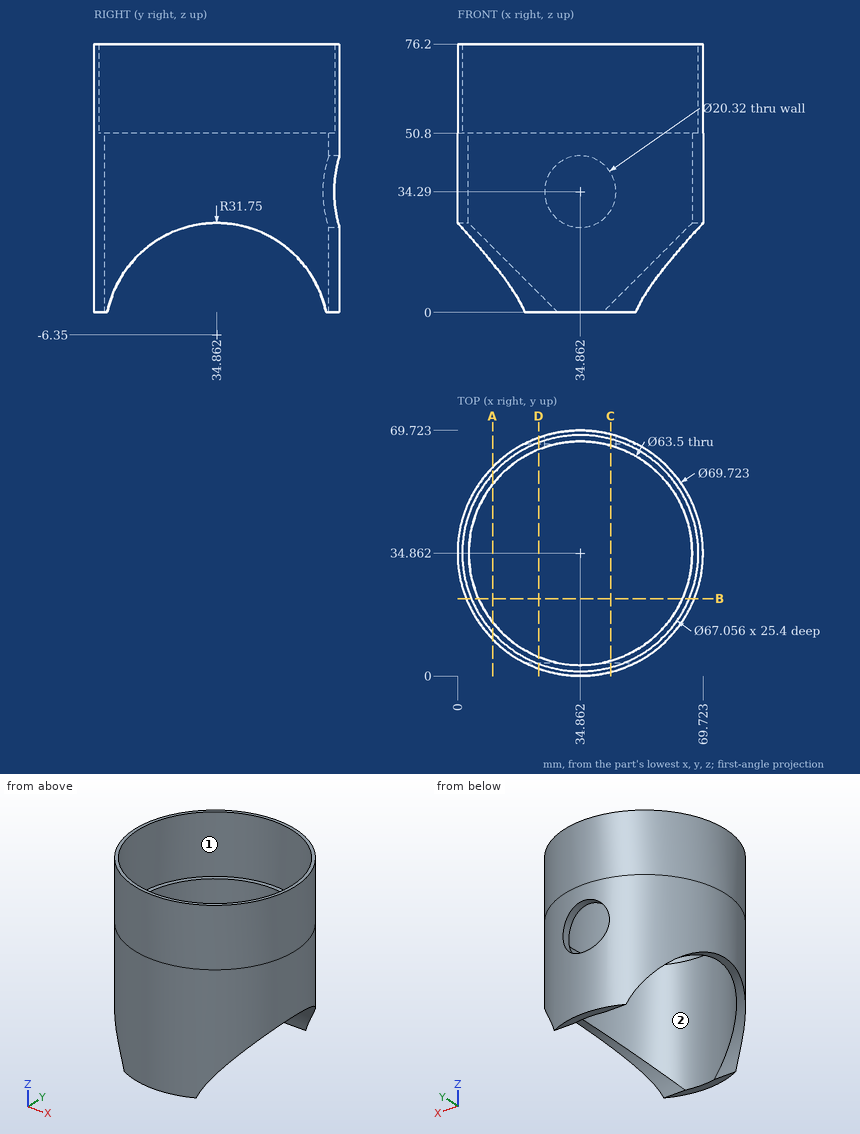
Source: three-view drawing plus pictorial views. Frame: mm from the lowest corner of the part. A direction names the side the tool comes from. Give positions to 0.01 mm unless a question says otherwise; leave off trailing zeros. Order: outer loops, then holes, each group sorted by start corner. A loop starts at its lowest first (then second) coordinate and runs counter-clockwise, first axis right, second up. Notation, with made-up numbers: (39, -37.5) - (88, -37.5) arc R29 ccw to (88, -14.5) - close; hole circle Ø5 at (23, 33). An arc over 180 degrees is marked (long way). Answer as a JSON object with one key per item and string values. Group by question number.
Q1. Set-up query: the marked faces 1 and 2. Return all of +Z, -Z, +X, -X, +Y, -Y with unobstructed straight access to the full face (end or side cutting, diameter ignored); none if empty.
Q2. Cut plane A-A, the plane x = 10. Output: boundary loops of the cut face in (y, z).
Q3. First-contact query: pin 1 Ø10 at (x, z) = (17, 18) entering from -Y; pin 2 Ø5 at (y, z) = (48.5, 42) entering from -X; pin 3 Ø12 at (x, z) = (34.86, 34.29) entering from -Y. Flat tips, straight axial feed; report the tip coordinate or a pass-through.
Q4. Cut plane D-D, the plane x = 23. Output: boundary loops of the cut face in (y, z).
Q5. Cut plane C-C, the plane x = 43.5. Count the separate pieces of the cut face and the enclosed holes in it.
Q6. Line query: probe 1 along X at (y, z) = (53.5, 63.5); probe 2 along Y at (x, z) = (35.5, 18) (1 decimal); probe 3 along X at (y, z) = (54.5, 43) (1 decimal). Output: solid intervals per line, ascending.
Q7. Cut plane B-B, the plane y = 22. Output: boundary loops of the cut face in (x, z) (1 decimal).
Results:
{
 "1": {"face 1": "+Z", "face 2": "+Z, -Z"},
 "2": {"outline": "(10.42, 13.92) arc R31.75 cw to (15.11, 18.51) - (15.11, 50.8) - (12.37, 50.8) - (12.37, 76.2) - (10.42, 76.2) - close; (54.61, 18.51) arc R31.75 cw to (59.3, 13.92) - (59.3, 76.2) - (57.36, 76.2) - (57.36, 50.8) - (54.61, 50.8) - close"},
 "3": {"pin 1": "y = 2.46", "pin 2": "x = 1.83", "pin 3": "y = 0"},
 "4": {"outline": "(2.08, 0) - (3.75, 0) arc R31.75 cw to (5.41, 5.51) - (5.41, 50.8) - (3.5, 50.8) - (3.5, 76.2) - (2.08, 76.2) - close; (64.31, 5.51) arc R31.75 cw to (65.97, 0) - (67.64, 0) - (67.64, 76.2) - (66.22, 76.2) - (66.22, 50.8) - (64.31, 50.8) - close"},
 "5": {"separate pieces": "3", "enclosed holes": "0"},
 "6": {"probe 1": "5.4 to 6.99, 62.73 to 64.32", "probe 2": "0 to 3.1, 66.6 to 69.7", "probe 3": "6.1 to 9.9, 59.8 to 63.7"},
 "7": {"outline": "(2.5, 22.7) - (5.8, 22.7) - (5.8, 50.8) - (3.9, 50.8) - (3.9, 76.2) - (2.5, 76.2) - close; (63.9, 22.7) - (67.3, 22.7) - (67.3, 76.2) - (65.8, 76.2) - (65.8, 50.8) - (63.9, 50.8) - close"}
}
